Design review of the part built by this model. Coordinates are the model's own, in mm. A direction names the side the tool comes from. Coordinates: 2 decimals unless noted, no trailing zeros. Loops run counter-clockwise (first coordinate to the right, second up) from the corner with the lowest first, then second, coordinate; pieces in that order, holes last. Notation, with made-up numbers: M 61,-12 L 69,-12 A20 cw 69,20 Z; hole C -1,38 d5. An arc over 180 degrees is marked long. Answer as a JSON object with one key per item and string values. Group by question number.
1. Insertion check: pin 1 (10 mm diameter, centred on x = -2, z = -47.5, fed in from +Y); pin 2 (2 mm diameter, centred on x = -13, y = 12.5, fed in from +Z); pin 3 (1 mm diameter, centred on y = -7, z = -6, fed in from -X); pin 4 (1 mm diameter, centred on y = 10, z = -118.5, fed in from -X). Each pin has a flat end and moves straight along its axis. Give the tip position at first contact, or say it passes through.
2. To check wall thickness, follow probe 1 along Z at (x, y) = (14.5, -5); probe 2 along X at (y, z) = (-1, -26); probe 3 along Y at (x, z) = (0, -43). State the ranges of each line that lie inside material, in increasing order.
3. Consider section B-B (z = -5). State the section outline as (x, y) points.
4. Machinability: for faces 1 (the cylindrical face through (13.66, -7.73, 13.7)), 2 (the flat face through (11.3, 0.2, 0)), which of the approach directions +Z, -Z, +X, -X, +Y, -Y give a long, thin tool a straight path to every point of the face, cutting with its end or side? Answer none if there is none.
5. Consider section C-C (z = -134). State the section outline as (x, y) points, then the cut area to 3 significant figures.
6. Consider section A-A (x = 0). State the section outline as (y, z) points, then the cut area to 3 significant figures.
from build123d import *

# Parameters (mm, degrees)
EXTRUDE_1_DEPTH = 14
SKETCH_3_R      = 11
EXTRUDE_2_DEPTH = 100
SKETCH_4_R      = 10.95
EXTRUDE_4_DEPTH = 50
FILLET_2_R      = 1


with BuildPart() as part:
    # 草图2 → 拉伸1 (new body)
    with BuildSketch(Plane.XY):
        Polygon((9.225, -15.9781687), (18.45, 0), (9.225, 15.9781687), (-9.225, 15.9781687), (-18.45, 0), (-9.225, -15.9781687), align=None)
    extrude(amount=EXTRUDE_1_DEPTH)

    # 草图3 → 拉伸2 (add)
    with BuildSketch(Plane(origin=(0, 0, 0), x_dir=(-1, 0, 0), z_dir=(0, 0, -1))):
        with Locations(Location((0, 0, 0), (0, 0, 180))):
            Circle(SKETCH_3_R)
    extrude(amount=EXTRUDE_2_DEPTH)

    # 草图4 → 拉伸4 (add)
    with BuildSketch(Plane(origin=(0, 0, -100), x_dir=(-1, 0, 0), z_dir=(0, 0, -1))):
        Circle(SKETCH_4_R)
    extrude(amount=EXTRUDE_4_DEPTH)

    # 圆角2
    fillet_2_edges = [part.edges().sort_by_distance(p)[0] for p in [
        (13.8375, 7.98908435, 14),
        (0, 15.9781687, 14),
        (-13.8375, 7.98908435, 14),
        (-13.8375, -7.98908435, 14),
        (10.95, 0, -150),
        (0, -15.9781687, 14),
        (-13.8375, -7.98908435, 0),
        (-13.8375, 7.98908435, 0),
        (0, 15.9781687, 0),
        (13.8375, -7.98908435, 14),
        (13.8375, 7.98908435, 0),
        (13.8375, -7.98908435, 0),
        (0, -15.9781687, 0),
    ]]
    fillet(fillet_2_edges, radius=FILLET_2_R)


solid = part.part
Findings below:
{
 "1": {"pin 1": "stops at y = 11", "pin 2": "passes through", "pin 3": "stops at x = -8.87", "pin 4": "stops at x = -5.45"},
 "2": {"probe 1": "z = 0 to 14", "probe 2": "x = -10.95 to 10.95", "probe 3": "y = -11 to 11"},
 "3": {"outline": "C 0,0 d22"},
 "4": {"face 1": "+Z, +X, -Y", "face 2": "-Z"},
 "5": {"outline": "C 0,0 d21.9", "area": "377 mm^2"},
 "6": {"outline": "M -15.98,1 A1 ccw -14.98,0 L -11,0 L -11,-100 L -10.95,-100 L -10.95,-149 A1 ccw -9.95,-150 L 9.95,-150 A1 ccw 10.95,-149 L 10.95,-100 L 11,-100 L 11,0 L 14.98,0 A1 ccw 15.98,1 L 15.98,13 A1 ccw 14.98,14 L -14.98,14 A1 ccw -15.98,13 Z", "area": "3,740 mm^2"}
}
